The model under review builds one solid part; all positions refer to its coordinate system, in mm. A direction names the side the tool comes from. Coordinates: 2 decimals unless noted, no trailing zeros. Loops run counter-clockwise (first coordinate to the right, second up) from the corner with the lowest first, then second, coordinate; pieces in that order, holes last. Notation, with made-up numbers: M -32.75,-1 L -19.75,-1 A33 ccw -19.75,32 Z; hole C 0.25,86 d11. An arc over 180 degrees is marked long. Return JSON: item names as keys, results as strings.
```python
from build123d import *

# Parameters (mm, degrees)
SKETCH_1_W          = 40.5
SKETCH_1_H          = 12
EXTRUDE_1_DEPTH     = 3
SKETCH_2_R          = 2.5
EXTRUDE_2_DEPTH     = 15.25
SKETCH_3_R          = 2.4
CUT_EXTRUDE_1_DEPTH = 30.5
FILLET_1_R          = 10
SKETCH_4_R          = 3.5
CUT_EXTRUDE_2_DEPTH = 30.5


with BuildPart() as part:
    # 草图1 → 凸台-拉伸1 (new body)
    with BuildSketch(Plane.XY):
        Rectangle(SKETCH_1_W, SKETCH_1_H)
    extrude(amount=EXTRUDE_1_DEPTH)

    # 草图2 → 凸台-拉伸2 (add, symmetric)
    with BuildSketch(Plane(origin=(0, 0, 0), x_dir=(0, 0, -1), z_dir=(1, 0, 0))):
        with BuildLine():
            Line((0, -6), (0, 14.75))
            ThreePointArc((0, 14.75), (-8.92202564, 20.78189786), (-11.195012861, 10.25479653))
            add(Edge.make_bspline(
                [(-3, -6), (-3, -3.834699913), (-2.949171736, 2.430786436), (-8.113125227, 7.035920639), (-11.195012861, 10.25479653)],
                knots=[0, 0, 0, 0, 0.319547367, 1, 1, 1, 1], degree=3))
            Line((-3, -6), (0, -6))
        make_face()
        with Locations(Location((-6.5, 14.75, 0), (0, 0, 180))):
            Circle(SKETCH_2_R, mode=Mode.SUBTRACT)
    extrude(amount=EXTRUDE_2_DEPTH, both=True)

    # 草图3 → 切除-拉伸1 (cut)
    with BuildSketch(Plane(origin=(0, 0, 0), x_dir=(-1, 0, 0), z_dir=(0, 0, -1))):
        with Locations((-8.9, 0.75)):
            Circle(SKETCH_3_R)
    cut_extrude_1 = extrude(amount=-CUT_EXTRUDE_1_DEPTH, mode=Mode.SUBTRACT)

    # 镜向1: 切除-拉伸1 across plane
    add(cut_extrude_1.mirror(Plane(origin=(0, 0, 0), x_dir=(0, 0, 1), z_dir=(1, 0, 0))), mode=Mode.SUBTRACT)

    # 圆角1
    # the kernel refuses this fillet: 10 mm, written as the material it takes off along each edge
    with BuildSketch(Plane(origin=(20.25, -6, -25), x_dir=(-1, 0, 0), z_dir=(0, 0, 1)), Plane(origin=(-20.25, -6, -25), x_dir=(0, 1, 0), z_dir=(0, 0, 1))) as fillet_1_piece_1:
        with BuildLine():
            CenterArc((FILLET_1_R, -FILLET_1_R), FILLET_1_R, 90, 90)
            Line((0, -FILLET_1_R), (0, 0))
            Line((0, 0), (FILLET_1_R, 0))
        make_face()
    extrude(amount=53, mode=Mode.SUBTRACT)

    # 草图4 → 切除-拉伸2 (cut)
    with BuildSketch(Plane.XY.offset(3)):
        with Locations(Location((-8.9, 0.75, 0), (0, 0, 180))):
            Circle(SKETCH_4_R)
    cut_extrude_2 = extrude(amount=CUT_EXTRUDE_2_DEPTH, mode=Mode.SUBTRACT)

    # 镜向2: 切除-拉伸2 across plane
    add(cut_extrude_2.mirror(Plane(origin=(0, 0, 0), x_dir=(0, 0, 1), z_dir=(1, 0, 0))), mode=Mode.SUBTRACT)


solid = part.part
```
1. Add section D-D on z = 11.75. Give the boundary of the cut face in (x, y).
Check values:
{"outline": "M -15.25,10.92 L 15.25,10.92 L 15.25,18.58 L -15.25,18.58 Z"}
2. Machinability: for faces 4 (the face through (-18, 6, 1)), 5 (the face through (-17, 2, 3)), 6 (the face through (10, -2, 3)), which of the approach directions +Z, -Z, +X, -X, +Y, -Y give a long, thin tool a straight path to every point of the face, cutting with its end or side? Answer none if there is none.
Check values:
{"face 4": "+Z, -Z, -X, +Y", "face 5": "+Z, -X, +Y, -Y", "face 6": "+Z"}
3. To check wall thickness, follow line 1 (X direction, y = 1.75, z = 2.5); line 2 (X direction, y = 7, z = 2); line 3 (Z direction, x = 6.5, y = -1). State the ranges of each line that lie inside material, in increasing order.
Check values:
{"line 1": "-19.99 to -11.08, -6.72 to 6.72, 11.08 to 19.99", "line 2": "-15.25 to 15.25", "line 3": "0 to 3"}
4. Add section A-A on z = 1.25. Give the boundary of the cut face in (x, y), plus the area to 3 significant figures.
Check values:
{"outline": "M -20.25,4 A10 ccw -10.25,-6 L 10.25,-6 A10 ccw 20.25,4 L 20.25,6 L 15.25,6 L 15.25,18.58 L -15.25,18.58 L -15.25,6 L -20.25,6 Z; hole C -8.9,0.75 d4.8; hole C 8.9,0.75 d4.8", "area": "791 mm²"}
5. The part is to be moulded in two halves that separate along Z. For faces 1 (the face through (0, 4, 0)), 2 (the face through (-0.21, 15.71, 8.81)), 3 (the face through (18, 6, 1)), say which applies: released by +Z, released by -Z, zero draft, split by the parting line, or undercut.
Check values:
{"face 1": "released by -Z", "face 2": "undercut", "face 3": "zero draft"}
6. Add section B-B on x = 8.9. State how many separate pieces and enclosed holes the cut face has, plus the area to 3 significant figures.
Check values:
{"separate pieces": "2", "enclosed holes": "1", "area": "169 mm²"}
7. Insertion check: pin 1 Ø4.5 at (x, y) = (8.9, 0.75) entering from +Z; pin 2 Ø6 at (y, z) = (12.5, 8) entering from -X; pin 3 Ø1.5 at (x, z) = (18, 1.5) entering from +Y; pin 4 Ø8 at (x, y) = (8.9, 0.75) entering from +Z. Each pin has a flat end and moves straight along its axis. Give the tip position at first contact, or say it passes through.
Check values:
{"pin 1": "through", "pin 2": "x = -15.25", "pin 3": "y = 6", "pin 4": "z = 6.09"}
